The drawing under review shows one solid part. Ordinate dimensions are in mm from its lowest x, y, z. A direction names the side the tool comes from. Coordinates: 2 decimals unless noted, no trailing zeros. Write each loop counter-clockwise with the first axis right and the second up, starting at its lowest first coordinate (ties: lowest second). Pieces come first, ordered by that corner, then holes. Notation, with made-up numbers: (-21, 65.5) -> (-9, 65.5) arc R34 ccw to (-9, 99.5) -> close; hole circle Ø10 at (-18, 71.25). An arc over 180 degrees is marked (long way). One line per item, written item: value. Start each with the question number.
1) For pin 1 Ø3 at (x, y) = (40, 10) entering from +Z; pin 2 Ø1.5 at (x, z) = (30, 2) entering from -Y; pin 3 Ø5 at (x, y) = (10, 11) entering from +Z; pin 4 Ø6 at (x, y) = (34.5, 4) entering from -Z, all flat-tipped, find the tip position at first contact; note any pin that passes through.
2) Add section B-B (x = 25). State the section outline as (y, z) points.
3) For probe 1 along X at (y, z) = (10, 6.5); probe 2 along Y at (x, z) = (10, 8.6); probe 3 along X at (y, z) = (9.5, 8.25), list the stretches that pass through material, from the lowest coordinate up. Write a range as from..to.
4) Add section A-A (y = 10). State the section outline as (x, z) points.
5) Add section C-C (z = 2). State the section outline as (x, y) points.
6) Machinability: for the marked faces 1, 2, 3, 4 and 5, which of the approach directions +Z, -Z, +X, -X, +Y, -Y give a long, thin tool a straight path to every point of the face, cutting with its end or side? Answer none if there is none.
7) Add section D-D (z = 5.5). State the section outline as (x, y) points.
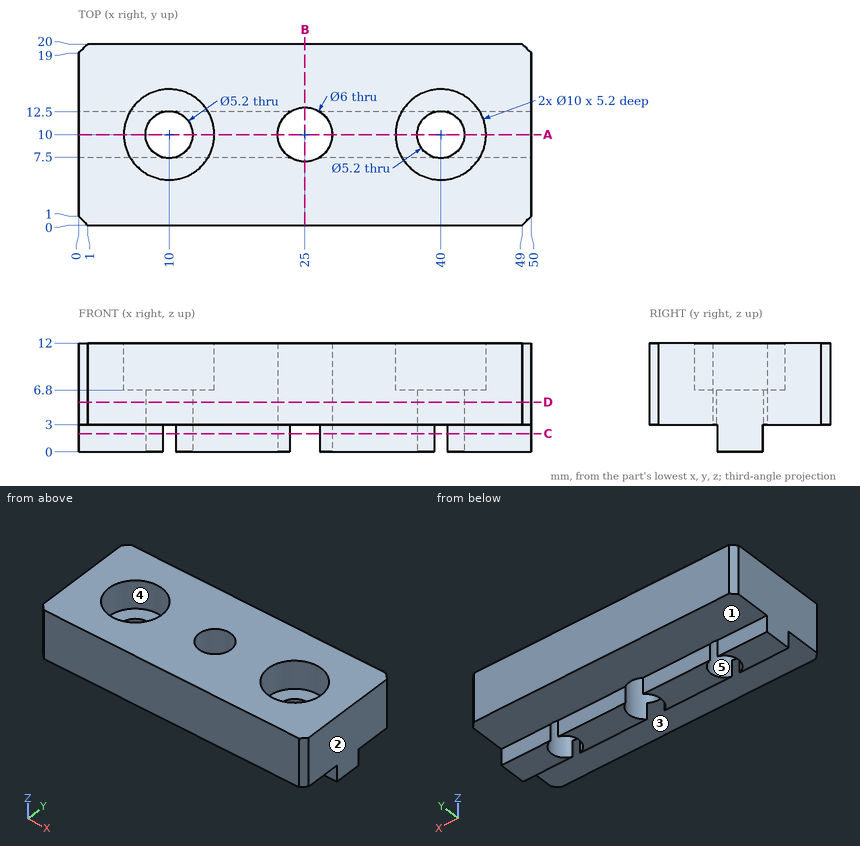
Numbers:
1. pin 1: through
1. pin 2: y = 7.5
1. pin 3: z = 6.8
1. pin 4: z = 3
2. outline: (0, 3) -> (7, 3) -> (7, 12) -> (0, 12) -> close; (13, 3) -> (20, 3) -> (20, 12) -> (13, 12) -> close
3. probe 1: 0..7.4, 12.6..22, 28..37.4, 42.6..50
3. probe 2: 0..5, 15..20
3. probe 3: 0..5.03, 14.97..22.04, 27.96..35.03, 44.97..50
4. outline: (0, 0) -> (7.4, 0) -> (7.4, 6.8) -> (5, 6.8) -> (5, 12) -> (0, 12) -> close; (12.6, 0) -> (22, 0) -> (22, 12) -> (15, 12) -> (15, 6.8) -> (12.6, 6.8) -> close; (28, 0) -> (37.4, 0) -> (37.4, 6.8) -> (35, 6.8) -> (35, 12) -> (28, 12) -> close; (42.6, 0) -> (50, 0) -> (50, 12) -> (45, 12) -> (45, 6.8) -> (42.6, 6.8) -> close
5. outline: (0, 7.5) -> (9.29, 7.5) arc R2.6 cw to (9.29, 12.5) -> (0, 12.5) -> close; (10.71, 7.5) -> (23.34, 7.5) arc R3 cw to (23.34, 12.5) -> (10.71, 12.5) arc R2.6 cw to start; (26.66, 7.5) -> (39.29, 7.5) arc R2.6 cw to (39.29, 12.5) -> (26.66, 12.5) arc R3 cw to start; (40.71, 7.5) -> (50, 7.5) -> (50, 12.5) -> (40.71, 12.5) arc R2.6 cw to start
6. face 1: -Z, +X, -X, +Y
6. face 2: +Z, -Z, +X, +Y, -Y
6. face 3: -Z, +X, -X, -Y
6. face 4: +Z
6. face 5: +Z, -Z
7. outline: (0, 1) -> (1, 0) -> (49, 0) -> (50, 1) -> (50, 19) -> (49, 20) -> (1, 20) -> (0, 19) -> close; hole circle Ø5.2 at (10, 10); hole circle Ø6 at (25, 10); hole circle Ø5.2 at (40, 10)
